Work out the finished part from the listing and answer in its coordinate system (mm). A direction names the side the tool comes from. Coordinates: 2 decimals unless noted, no trailing zeros. Write each loop counter-clockwise with the first axis right and the second up, starting at its lowest first coordinate (ties: lowest second). Pieces come first, ordered by that corner, then holes. Notation, with made-up numbers: M 67.25,59 L 78.25,59 A17 cw 78.25,72 Z; hole C -28,5 d4. An arc over 180 degrees is marked long. Answer as CSV lines item,"result". Start each with the question number.
(1) The mould has two halves that part along X. Classify faces 1 (the flat face through (75, 5, 0)), 2 (the flat face through (63, 5, -22)), 3 (the flat face through (68, 5, -1)), 4 (the flat face through (-14, 5, 14.5)): released by +X, released by -X, zero draft, split by the parting line, or undercut.
(2) A cutting plane is placed at A-A on z = 0. Give the vertices of the cut face in (x, y), then the cut area to 3 significant figures.
(3) A flat-ended cylindrical pin translates along its axis: P1, Ø1, axis at x = 58, z = -8, coming from the -Y side. Find the tip coordinate at first contact, or state that the pin passes through.
(4) A cutting plane is placed at D-D on z = 18. Give the vertices of the cut face in (x, y), then the cut area to 3 significant figures.
(5) A cutting plane is placed at B-B on x = 14. Give the vertices of the cut face in (y, z).
(6) A cutting plane is placed at C-C on y = 8. Give the vertices of the cut face in (x, z), then the cut area to 3 significant figures.
(7) Find the intervals of material crossed by L1, parallel to X at y = 7.5, z = 0; L2, parallel to Z at x = -61.5, y = 5; L3, parallel to X at y = 9, z = -15, in increasing order. Write a range as [from, to].
(8) For faces 5 (the flat face through (58, 5, -1)), 6 (the flat face through (-14, 5, -14.5)), 7 (the flat face through (-75, 5, 20)), determine the directions among +Z, -Z, +X, -X, +Y, -Y from which every point of the face is accessible in a straight line to the end or side of a thin tool.
from build123d import *

# Parameters (mm, degrees)
SKETCH1_W           = 150
SKETCH1_H           = 51
BOSS_EXTRUDE1_DEPTH = 10
SKETCH2_W           = 10
SKETCH2_H           = 42
CUT_EXTRUDE1_DEPTH  = 80.845162659
SKETCH3_W           = 123
SKETCH3_H           = 29
CUT_EXTRUDE2_DEPTH  = 80.845162659
SKETCH4_R           = 2
CUT_EXTRUDE3_DEPTH  = 80.845162659


with BuildPart() as part:
    # Sketch1 → Boss-Extrude1 (new body)
    with BuildSketch(Plane(origin=(0, 0, 0), x_dir=(1, 0, 0), z_dir=(0, 1, 0))):
        Rectangle(SKETCH1_W, SKETCH1_H)
    extrude(amount=BOSS_EXTRUDE1_DEPTH)

    # Sketch2 → Cut-Extrude1 (cut, through all)
    with BuildSketch(Plane(origin=(0, 10, 0), x_dir=(1, 0, 0), z_dir=(0, 1, 0))):
        with Locations((63, 1)):
            Rectangle(SKETCH2_W, SKETCH2_H)
    extrude(amount=-CUT_EXTRUDE1_DEPTH, mode=Mode.SUBTRACT)

    # Sketch3 → Cut-Extrude2 (cut, through all)
    with BuildSketch(Plane(origin=(0, 10, 0), x_dir=(1, 0, 0), z_dir=(0, 1, 0))):
        with Locations((-13.5, 0)):
            Rectangle(SKETCH3_W, SKETCH3_H)
    extrude(amount=-CUT_EXTRUDE2_DEPTH, mode=Mode.SUBTRACT)

    # Sketch4 → Cut-Extrude3 (cut, through all)
    with BuildSketch(Plane(origin=(0, 10, 0), x_dir=(1, 0, 0), z_dir=(0, 1, 0))):
        with Locations(Location((72, 0, 0), (0, 0, 270))):
            Circle(SKETCH4_R)
    extrude(amount=-CUT_EXTRUDE3_DEPTH, mode=Mode.SUBTRACT)


solid = part.part
Here are the results:
1,face 1,"released by +X"
1,face 2,"undercut"
1,face 3,"undercut"
1,face 4,"zero draft"
2,outline,"M 48,0 L 58,0 L 58,10 L 48,10 Z; M 68,0 L 70,0 L 70,10 L 68,10 Z; M 74,0 L 75,0 L 75,10 L 74,10 Z"
2,area,"130 mm^2"
3,P1,"stops at y = 0"
4,outline,"M -75,0 L 58,0 L 58,10 L -75,10 Z; M 68,0 L 75,0 L 75,10 L 68,10 Z"
4,area,"1,400 mm^2"
5,outline,"M 0,-25.5 L 10,-25.5 L 10,-14.5 L 0,-14.5 Z; M 0,14.5 L 10,14.5 L 10,25.5 L 0,25.5 Z"
6,outline,"M -75,-25.5 L 75,-25.5 L 75,25.5 L -75,25.5 L -75,14.5 L 48,14.5 L 48,-14.5 L -75,-14.5 Z; hole M 58,-22 L 68,-22 L 68,20 L 58,20 Z; hole C 72,0 d4"
6,area,"3,650 mm^2"
7,L1,"x = [48, 58], [68, 70], [74, 75]"
7,L2,"z = [-25.5, -14.5], [14.5, 25.5]"
7,L3,"x = [-75, 58], [68, 75]"
8,face 5,"+Y, -Y"
8,face 6,"-X, +Y, -Y"
8,face 7,"+Z, -Z, -X, +Y, -Y"
